Geometry check sheet. Reference: the model listing, model coordinates, mm. Coordinates: 2 decimals unless noted, no trailing zeros. Write each loop counter-clockwise with the first axis right and the second up, starting at its lowest first coordinate (ties: lowest second). Pieces come first, ordered by that corner, then holes. Notation, with made-up numbers: M -2.75,-36.5 L 34.25,-36.5 A20 cw 34.25,2.5 Z; hole C 76,-33.75 d11. An arc over 180 degrees is marked long. Answer as a JSON object with one key per item and string values. Group by question number.
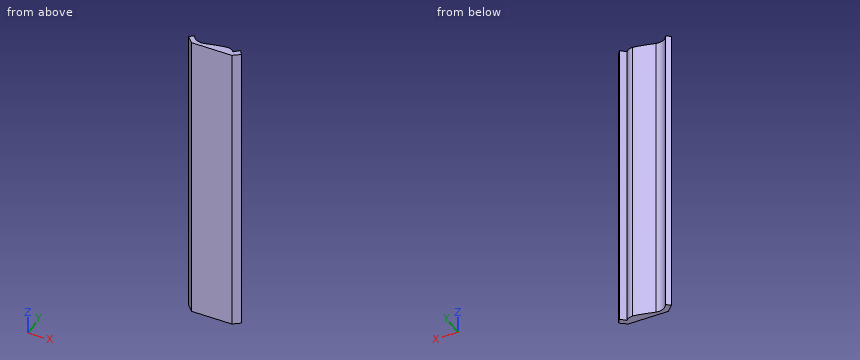
```python
from build123d import *

# Parameters (mm, degrees)
F1_DEPTH = 609.6


with BuildPart() as f1:
    # F0 (on Top) → F1 (new body)
    with BuildSketch(Plane.XY):
        with BuildLine():
            Line((-13.314313, 13.787375), (0, 0))
            Line((0, 0), (81.28, 0))
            Line((81.28, 0), (95.651687, 10.441642))
            Line((95.651687, 10.441642), (88.843723, 19.812))
            Line((88.843723, 19.812), (78.395705, 10.16))
            ThreePointArc((78.395705, 10.16), (71.810031, 15.310411), (63.653308, 17.145))
            add(Edge.make_bspline(
                [(20.882963, 8.157931), (28.513048, 9.843092), (53.867209, 17.145), (63.653308, 17.145)],
                knots=[0, 0, 0, 0, 43.704346, 43.704346, 43.704346, 43.704346], degree=3))
            ThreePointArc((20.882963, 8.157931), (6.341194, 9.738896), (-4.265176, 19.812))
            Line((-4.265176, 19.812), (-13.314313, 13.787375))
        make_face()
    extrude(amount=F1_DEPTH)


solid = f1.part
```
1) Section check A-A (x = 71). Record the cut outline in (y, z).
2) Material ranges on probe 1 along Y at (x, z) = (74.5, 452); probe 2 along Y at (x, z) = (73, 328.5); probe 3 along X at (y, z) = (4.5, 243.5), recorded low to high. Write a range as [from, to].
3) Section check B-B (y = 4). Record the cut outline in (x, z).
4) Go/stop test with flat-tipped pins: pin 1 Ø5 at (y, z) = (17.5, 97.5) entering from +X; pin 2 Ø4 at (x, z) = (25.5, 183) entering from +Y; pin 3 Ø10 at (y, z) = (14, 232) entering from -X. Record where each tip stops, or that it passes through.
Entries:
{
 "1": {"outline": "M 0,0 L 15.67,0 L 15.67,609.6 L 0,609.6 Z"},
 "2": {"probe 1": "[0, 13.76]", "probe 2": "[0, 14.69]", "probe 3": "[-4.35, 87.47]"},
 "3": {"outline": "M -3.86,0 L 86.79,0 L 86.79,609.6 L -3.86,609.6 Z"},
 "4": {"pin 1": "x = 92.34", "pin 2": "y = 9.79", "pin 3": "x = -13.31"}
}
